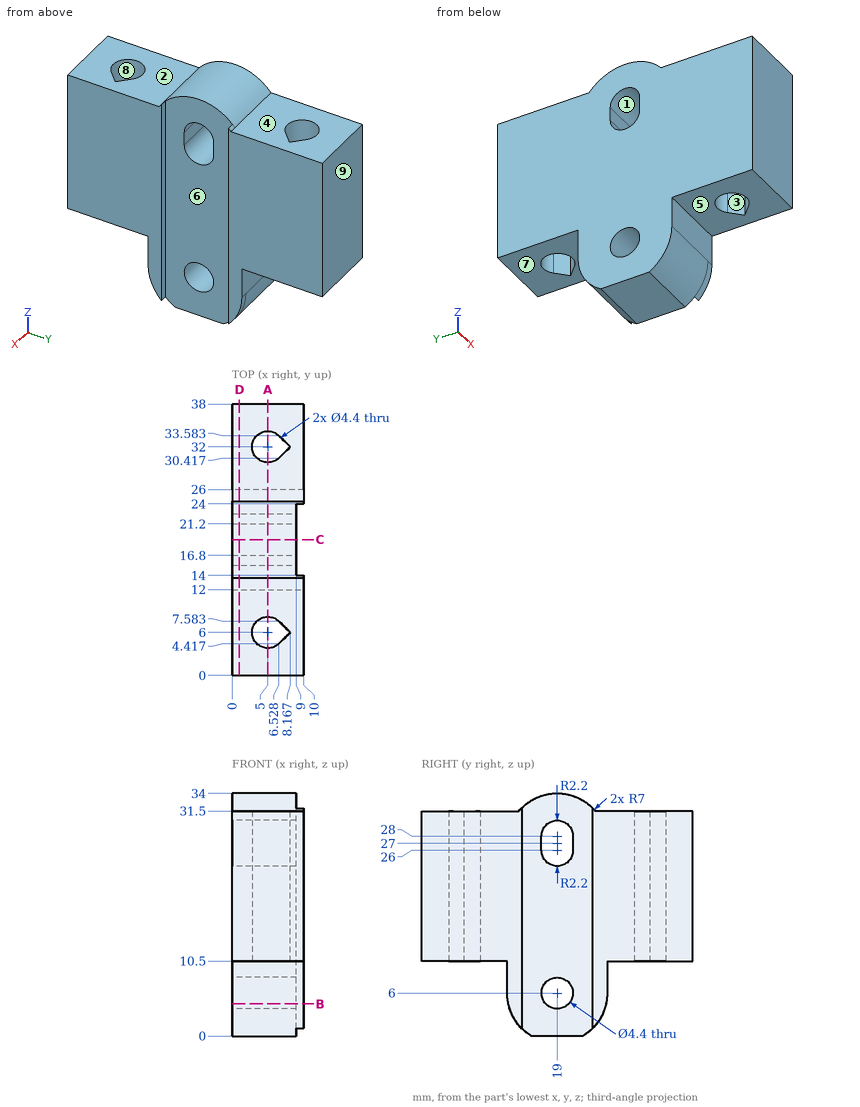
Input: dimensioned drawing with shaded views. Units: mm. Origin: part minimum x, y, z. A direction names the side the tool comes from. Coordinates: 2 decimals unless noted, no trailing zeros. Loops run counter-clockwise (first coordinate to the right, second up) from the corner with the lowest first, then second, coordinate; pieces in that order, holes last. Notation, with made-up numbers: (-31, 75) -> (19, 75) arc R8 ccw to (19, 87) -> close; hole circle Ø6 at (2, -17). An arc over 180 degrees is marked (long way). One line per item, written item: value. Start each with the question number.
Q1. Section query A-A, the plane x = 5. Return the cut outline in (y, z) (1 decimal).
Q2. Section query B-B, the plane z = 4.5. Return the cut outline in (x, y).
Q3. Set-up query: the marked faces 1, 2, 3, 4 and 5. Return all of +Z, -Z, +X, -X, +Y, -Y with unobstructed straight access to the full face (end or side cutting, diameter ignored); none if empty.
Q4. Section query D-D, the plane x = 1. Return the cut outline in (y, z) (1 decimal).
Q5. Mould query, pull axis Y, two halves, no side actions, for the marked faces 6, 7, 8 and 9. Classes: pulls with the +Y half, pulls with the -Y half, needs draft (parallel to the pull), parting line crosses it, or undercut.
Q6. Section query C-C, the plane y = 19. Return the cut outline in (x, z), and give its area (3 significant figures).
Q7. Contact query for flat-ended pins moving along their axis: P1, Ø5, axis at x = 5, y = 32, coming from the +Z side; P2, Ø3.5, axis at x = 5, y = 6, coming from the +Z side; P3, Ø1.3, axis at x = 2.5, z = 7.5, coming from the -Y side; P4, Ø5, axis at x = 4, y = 30, coming from the -Z side. Output: stop coordinate, or through.
Q8. Line query: line 1 along Y through (x, z) = (5, 18.75); line 2 along Y through (x, z) = (6, 26); line 3 along Y through (x, z) = (6.25, 6). Output: solid intervals per line, ascending.
Results:
1. outline: (0, 10.5) -> (3.8, 10.5) -> (3.8, 31.5) -> (0, 31.5) -> close; (8.2, 10.5) -> (12, 10.5) -> (12, 6) arc R7 ccw to (15.4, 0) -> (22.6, 0) arc R7 ccw to (26, 6) -> (26, 10.5) -> (29.8, 10.5) -> (29.8, 31.5) -> (24.4, 31.5) arc R7 ccw to (13.6, 31.5) -> (8.2, 31.5) -> close; (34.2, 10.5) -> (38, 10.5) -> (38, 31.5) -> (34.2, 31.5) -> close; hole circle Ø4.4 at (19, 6); hole (16.8, 26) arc R2.2 ccw to (21.2, 26) -> (21.2, 28) arc R2.2 ccw to (16.8, 28) -> close
2. outline: (0, 12.16) -> (10, 12.16) -> (10, 14) -> (9, 14) -> (9, 17.39) -> (0, 17.39) -> close; (0, 20.61) -> (9, 20.61) -> (9, 24) -> (10, 24) -> (10, 25.84) -> (0, 25.84) -> close
3. face 1: +X, -X
3. face 2: +Z, +X, -X, -Y
3. face 3: +Z, -Z
3. face 4: +Z, +X, -X, +Y
3. face 5: -Z, +X, -X, -Y
4. outline: (0, 10.5) -> (12, 10.5) -> (12, 6) arc R7 ccw to (15.4, 0) -> (22.6, 0) arc R7 ccw to (26, 6) -> (26, 10.5) -> (38, 10.5) -> (38, 31.5) -> (24.4, 31.5) arc R7 ccw to (13.6, 31.5) -> (0, 31.5) -> close; hole circle Ø4.4 at (19, 6); hole (16.8, 26) arc R2.2 ccw to (21.2, 26) -> (21.2, 28) arc R2.2 ccw to (16.8, 28) -> close
5. face 6: undercut
5. face 7: needs draft
5. face 8: undercut
5. face 9: pulls with the +Y half
6. outline: (0, 0) -> (9, 0) -> (9, 3.8) -> (0, 3.8) -> close; (0, 8.2) -> (9, 8.2) -> (9, 23.8) -> (0, 23.8) -> close; (0, 30.2) -> (9, 30.2) -> (9, 34) -> (0, 34) -> close
6. area: 209 mm^2
7. P1: z = 31.5
7. P2: through
7. P3: y = 12
7. P4: z = 10.5
8. line 1: 0 to 3.8, 8.2 to 29.8, 34.2 to 38
8. line 2: 0 to 4.04, 7.96 to 16.8, 21.2 to 30.04, 33.96 to 38
8. line 3: 12 to 16.8, 21.2 to 26
